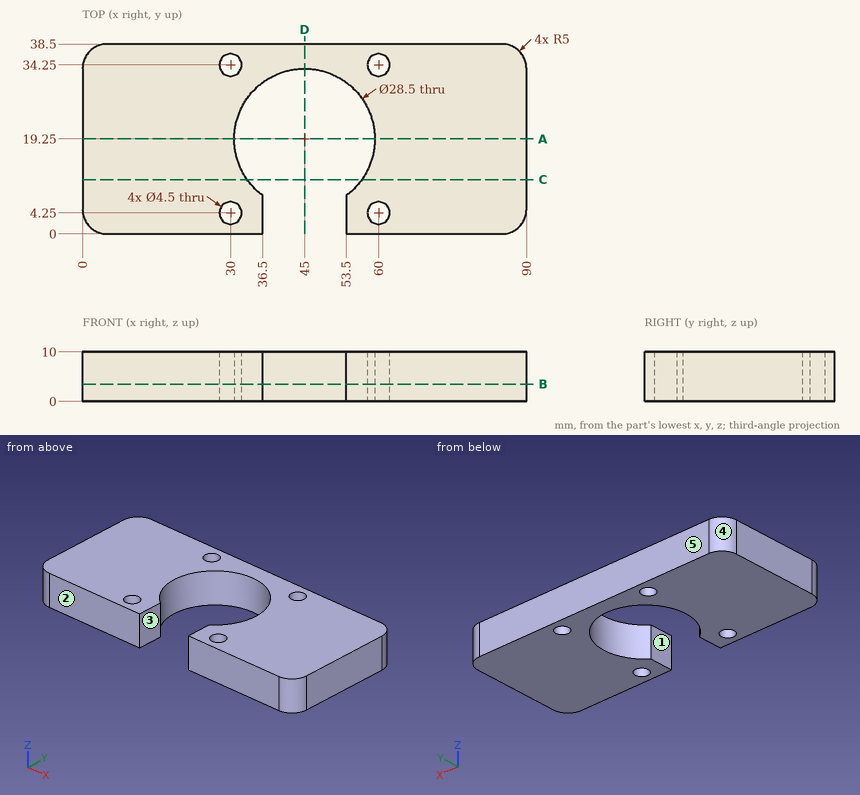
Verification items for this drawing (mm, ordinates from the low corner). A direction names the side the tool comes from. Give positions to 0.01 mm unless a question says otherwise; leave off trailing zeros. Loops run counter-clockwise (first coordinate to the right, second up) from the corner with the lowest first, then second, coordinate; pieces in that order, holes last. Notation, with made-up numbers: M 59,67 L 79,67 A10 cw 79,71 Z; hole C 29,86 d8. An arc over 180 degrees is marked long. Answer as CSV lines item,"result".
Item 1: Access from +Z, -Z, +X, -X, +Y, -Y to the whole of each face (thin tool, end or side, straight path). Record for the marked faces 1 and 2.
Values:
face 1,"+Z, -Z, -Y"
face 2,"+Z, -Z, +X, -X, -Y"
Item 2: Cross-section at D-D on x = 45. Record the cut outline in (y, z), and give its area (3 significant figures).
Values:
outline,"M 33.5,0 L 38.5,0 L 38.5,10 L 33.5,10 Z"
area,"50.0 mm²"
Item 3: Release check for a two-part mould opening along X. For the marked faces 3, 4 and 5 record: pulls with the +X half, pulls with the -X half, needs draft (parallel to the pull), parting line crosses it, or undercut.
Values:
face 3,"undercut"
face 4,"pulls with the -X half"
face 5,"needs draft"
Item 4: Depth check by flat-ended pin: P1, Ø4, axis at x = 60, y = 34.25, coming from the -Z side. Enter the tip coordinate at first touch or a pass-through.
Values:
P1,"passes through"
Item 5: Cross-section at B-B on z = 3.5. Record the cut outline in (x, y).
Values:
outline,"M 0,5 A5 ccw 5,0 L 36.5,0 L 36.5,7.81 A14.25 cw long 53.5,7.81 L 53.5,0 L 85,0 A5 ccw 90,5 L 90,33.5 A5 ccw 85,38.5 L 5,38.5 A5 ccw 0,33.5 Z; hole C 30,4.25 d4.5; hole C 30,34.25 d4.5; hole C 60,4.25 d4.5; hole C 60,34.25 d4.5"
Item 6: Material ranges on line 1 (Y direction, x = 60, z = 5.5); line 2 (Y direction, x = 45, z = 7.5); line 3 (X direction, y = 24.5, z = 3), recorded low to high.
Values:
line 1,"y = 0 to 2, 6.5 to 32, 36.5 to 38.5"
line 2,"y = 33.5 to 38.5"
line 3,"x = 0 to 31.75, 58.25 to 90"
Item 7: Cross-section at A-A on y = 19.25. Record the cut outline in (x, z), and give its area (3 significant figures).
Values:
outline,"M 0,0 L 30.75,0 L 30.75,10 L 0,10 Z; M 59.25,0 L 90,0 L 90,10 L 59.25,10 Z"
area,"615 mm²"
Item 8: Cross-section at C-C on y = 11. Record the cut outline in (x, z).
Values:
outline,"M 0,0 L 33.38,0 L 33.38,10 L 0,10 Z; M 56.62,0 L 90,0 L 90,10 L 56.62,10 Z"
